Input: part model. Units: mm. Frame: model coordinates. Give positions to 0.01 mm unless a question says otherwise; leave off trailing zeros. Loops run counter-clockwise (first coordinate to the right, second up) from the corner with the lowest first, then second, coordinate; pieces in that order, holes last. Notation, with made-up numbers: M -9,21 L 8,21 A18 cw 8,43 Z; hole C 11,-9.75 d4. An arc over 180 degrees is marked long. Use a Markdown table: item, result. Add a question column.
from build123d import *

# Parameters (mm, degrees)
F2_R = 26.2509
F0_R = 30.1625
F5_R = 26.2509
F4_R = 22.3393


with BuildPart() as f3:
    # F2 (on offset) → F3 section 0
    with BuildSketch(Plane.XZ.offset(25.4)):
        Circle(F2_R)
    # F0 (on Front) → F3 section 1
    with BuildSketch(Plane.XZ):
        Circle(F0_R)
    loft()

    # F5 (on face) → F6 section 0
    with BuildSketch(Plane(origin=(0, 0, 0), x_dir=(-1, 0, 0), z_dir=(0, 1, 0))):
        Circle(F5_R)
    # F4 (on face) → F6 section 1
    with BuildSketch(Plane.XZ.offset(25.4)):
        Circle(F4_R)
    loft(mode=Mode.SUBTRACT)

    # F7: F3 across face


with BuildPart() as f3_1:
    add(f3.part)
    add(f3.part.mirror(Plane(origin=(0, 0, 0), x_dir=(-1, 0, 0), z_dir=(0, 1, 0))))


solid = f3_1.part
1) Pull-direction query (X, two-part tool) for faces 1 (the conical face through (-12.81, 15.7, 20.1)), 2 (the flat face through (-14, 25.4, 18)), 3 (the conical face through (-12.81, -15.7, 20.1)), 4 (the conical face through (-21.716, -18.167, -16.651)); classes: pulls with the +X half, pulls with the -X half, needs draft (parallel to the pull), parting line crosses it, or undercut.
2) Contact query for flat-ended pins moving along their axis: P1, Ø3, axis at x = 10, y = -11, coming from the +Z side; P2, Ø1.5, axis at x = -12, y = 14.5, coming from the -Z side; P3, Ø12, axis at x = 14, y = -3, coming from the -Z side. Output: stop coordinate, or through.
3) Section query C-C, the plane y = 17.5. Return the cut outline in (x, z) (1 decimal), and give its area (3 significant figures).
4) Section query B-B, the plane y = 5. Return the cut outline in (x, z) (1 decimal), and give its area (3 significant figures).
5) Ray query, line 1 (Z direction, x = -2, y = -6); line 2 (Z direction, x = 17, y = 19); line 3 (X direction, y = 16, z = -1). Return the intervals inside material, ascending. Write a range as [from, to].
6) Section query A-A, the plane x = 0. Return the cut outline in (y, z).
Entries:
| question | item | result |
|---|---|---|
| 1 | face 1 | undercut |
| 1 | face 2 | needs draft |
| 1 | face 3 | undercut |
| 1 | face 4 | parting line crosses it |
| 2 | P1 | stops at z = 27.23 |
| 2 | P2 | stops at z = -25.59 |
| 2 | P3 | stops at z = -28.85 |
| 3 | outline | C 0,0 d54.9; hole C 0,0 d47.1 |
| 3 | area | 627 mm² |
| 4 | outline | C 0,0 d58.8; hole C 0,0 d51 |
| 4 | area | 674 mm² |
| 5 | line 1 | z = [-29.17, -25.25], [25.25, 29.17] |
| 5 | line 2 | z = [-21.28, -15.97], [15.97, 21.28] |
| 5 | line 3 | x = [-27.68, -23.77], [23.77, 27.68] |
| 6 | outline | M -25.4,-26.25 L 0,-30.16 L 25.4,-26.25 L 25.4,-22.34 L 0,-26.25 L -25.4,-22.34 Z; M -25.4,22.34 L 0,26.25 L 25.4,22.34 L 25.4,26.25 L 0,30.16 L -25.4,26.25 Z |
